```python
from build123d import *

# Parameters (mm, degrees)
SKETCH2_R           = 10
SKETCH2_R_2         = 5
BOSS_EXTRUDE3_DEPTH = 10
SKETCH3_R           = 15
CUT_EXTRUDE1_DEPTH  = 5
SKETCH4_R           = 10
CUT_EXTRUDE2_DEPTH  = 259.488315973


with BuildPart() as part:
    # Sketch2 → Boss-Extrude3 (new body)
    with BuildSketch(Plane.XY):
        with BuildLine():
            Line((-207.050381934, 98.472297517), (-147.050381934, 98.472297517))
            ThreePointArc((-147.050381934, 98.472297517), (-142.656983652, 87.865695799), (-132.050381934, 83.472297517))
            Line((-132.050381934, 83.472297517), (-111.050381934, 83.472297517))
            ThreePointArc((-111.050381934, 83.472297517), (-91.050381934, 63.472297517), (-111.050381934, 43.472297517))
            Line((-111.050381934, 43.472297517), (-132.050406277, 43.472297517))
            ThreePointArc((-132.050406277, 43.472297517), (-142.656990782, 39.078906365), (-147.050381934, 28.47232186))
            Line((-147.050381934, 28.47232186), (-207.050381934, 28.47232186))
            ThreePointArc((-207.050381934, 28.47232186), (-238.944378708, 63.472309688), (-207.050381934, 98.472297517))
        make_face()
        with Locations((-111.050381934, 63.472297517)):
            Circle(SKETCH2_R, mode=Mode.SUBTRACT)
        with Locations((-159.050381934, 63.472309688)):
            Circle(SKETCH2_R_2, mode=Mode.SUBTRACT)
    extrude(amount=BOSS_EXTRUDE3_DEPTH)

    # Sketch3 → Cut-Extrude1 (cut)
    with BuildSketch(Plane.XY.offset(10)):
        with Locations((-203.793152693, 63.472309688)):
            Circle(SKETCH3_R)
    extrude(amount=-CUT_EXTRUDE1_DEPTH, mode=Mode.SUBTRACT)

    # Sketch4 → Cut-Extrude2 (cut, through all)
    with BuildSketch(Plane.XY.offset(5)):
        with Locations((-203.793152693, 63.472309688)):
            Circle(SKETCH4_R)
    extrude(amount=-CUT_EXTRUDE2_DEPTH, mode=Mode.SUBTRACT)


solid = part.part
```
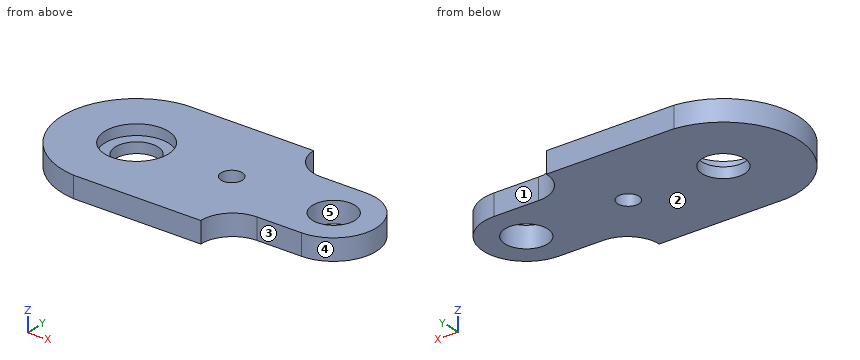
Geometry: final body of the model. Coordinates: model frame, mm. Face numbers are marked on the shaded views. A direction names the side the tool comes from. Give positions to 0.01 mm unless a question says otherwise; leave off trailing zeros. Loops run counter-clockwise (first coordinate to the right, second up) from the corner with the lowest first, then second, coordinate; pieces in that order, holes last. Notation, with made-up numbers: (64.25, 76.5) - (70.25, 76.5) arc R27 cw to (70.25, 99.5) - close; hole circle Ø4 at (-8, 53.25). An arc over 180 degrees is marked (long way). Answer as CSV lines item,"result". Start each with the question number.
(1) Section query B-B (y = 70). Output: boundary loops of the cut face in (x, z), and give its area (3 significant figures).
(2) Ray query, line 1 along X through (y, z) = (64.5, 8.5); line 2 along Y through (x, z) = (-123, 6); line 3 along X through (y, z) = (71.5, 5.75). Return the intervals inside material, ascending. Write a range as [from, to].
(3) Mould query, pull axis X, two halves, no side actions, for the marked faces 3, 4 and 5. Classes: +X half, -X half, draft (parallel to the pull), parting line (faces both ways), or undercut.
(4) Reachability of the marked faces 1 and 2 from +Z, -Z, +X, -X, +Y, -Y: full face, straight path, thin tool, end or side. Return the list, or none.
(5) Section query D-D (x = -118). Output: boundary loops of the cut face in (y, z).
(6) Pin query (flat end, axial travel): P1, Ø9, axis at x = -197, y = 67.5, coming from the +Z side; P2, Ø4, axis at y = 65, z = 4.5, coming from the -X side; P3, Ø6, axis at x = -130.5, z = 2.5, coming from the -Y side; P4, Ø16, axis at x = -111.05, y = 63.47, coming from the -Z side. Return the tip coordinate at first contact, or that it passes through.
(7) Section query C-C (z = 2). Output: boundary loops of the cut face in (x, y).
(8) Section query A-A (x = -200). Output: boundary loops of the cut face in (y, z), and give its area (3 significant figures).
Worked answers:
1,outline,"(-238.33, 0) - (-211.37, 0) - (-211.37, 5) - (-217.3, 5) - (-217.3, 10) - (-238.33, 10) - close; (-196.22, 0) - (-118.63, 0) - (-118.63, 10) - (-190.29, 10) - (-190.29, 5) - (-196.22, 5) - close; (-103.47, 0) - (-92.15, 0) - (-92.15, 10) - (-103.47, 10) - close"
1,area,"1,100 mm^2"
2,line 1,"x = [-238.93, -218.76], [-188.83, -163.94], [-154.16, -121], [-101.1, -91.08]"
2,line 2,"y = [43.47, 83.47]"
2,line 3,"x = [-238.02, -216.46], [-191.12, -117.01], [-105.09, -92.73]"
3,face 3,"draft"
3,face 4,"+X half"
3,face 5,"undercut"
4,face 1,"+Z, -Z, +X, +Y"
4,face 2,"-Z, +X, -X, +Y, -Y"
5,outline,"(43.47, 0) - (56.28, 0) - (56.28, 10) - (43.47, 10) - close; (70.66, 0) - (83.47, 0) - (83.47, 10) - (70.66, 10) - close"
6,P1,"stops at z = 5"
6,P2,"stops at x = -238.94"
6,P3,"stops at y = 43.4"
6,P4,"passes through"
7,outline,"(-207.05, 28.47) - (-147.05, 28.47) arc R15 cw to (-132.05, 43.47) - (-111.05, 43.47) arc R20 ccw to (-111.05, 83.47) - (-132.05, 83.47) arc R15 cw to (-147.05, 98.47) - (-207.05, 98.47) arc R35.15 ccw to start; hole circle Ø20 at (-203.79, 63.47); hole circle Ø10 at (-159.05, 63.47); hole circle Ø20 at (-111.05, 63.47)"
8,outline,"(28.47, 0) - (54.22, 0) - (54.22, 5) - (48.96, 5) - (48.96, 10) - (28.47, 10) - close; (72.72, 0) - (98.47, 0) - (98.47, 10) - (77.98, 10) - (77.98, 5) - (72.72, 5) - close"
8,area,"462 mm^2"
